Read the model definition and answer for the solid it produces. Units are mm, in the model's axes. A direction names the side the tool comes from. Coordinates: 2 decimals unless noted, no trailing zeros. Order: outer loops, then holes, each group sorted by start corner. A loop starts at its lowest first (then second) coordinate and runs counter-clockwise, first axis right, second up. Notation, with made-up numbers: (52.5, 0.5) -> (96.5, 0.5) arc R31 cw to (96.5, 31.5) -> close; hole circle Ø8 at (85, 46). An arc over 180 degrees is marked (long way). Answer as a JSON object with one key per item and string values. Group by question number.
1) Section B-B on y = 1 is taken. Determine the outline of the cut face in (x, z).
2) Section C-C on z = 0 is taken. Determine the outline of the cut face in (x, y), and give its area (3 significant figures).
3) Consider L1, parallel to Z at x = 0, y = 3.25; L2, parallel to Y at x = 3, z = -3; L3, parallel to X at y = 1.25, z = 5.5. Determine where each line is inside the solid, lowest interval first.
4) Determine the mould class of faces 3 (the cylindrical face through (3.47, 7.66, 15.62)), 4 (the cylindrical face through (-2.17, 4.56, -9.76)), 5 (the flat face through (0, 12, 0)) for opening direction X: released by +X, released by -X, zero draft, split by the parting line, or undercut.
5) Section D-D on y = 7.5 is taken. Determine the outline of the cut face in (x, z).
6) Section A-A on x = 0 is taken. Determine the outline of the cut face in (y, z).
7) A tool of negligible diameter and unlimited length cuts with its end or side. For faces 1 (the flat face through (-11, 5, 9)), 2 (the flat face through (-5.2, 0, 9.1)), from which of +Z, -Z, +X, -X, +Y, -Y can it reach the whole face along a straight path? Write none if from no direction.
8) Given pin 1 (1 mm diameter, centred on x = -2, y = 3, fed in from +Z); pin 2 (6 mm diameter, centred on x = 1.5, y = 3.5, fed in from -Z); pin 3 (4 mm diameter, centred on y = 2.5, z = 1.5, fed in from -X); pin 4 (1 mm diameter, centred on y = 8, z = 10, fed in from +X), each flat-ended and moving along its own axis, determine where each tip first touches the part or whether it passes through.
from build123d import *

# Parameters (mm, degrees)
FILLET1_R          = 2
SKETCH2_R          = 10
CUT_EXTRUDE1_DEPTH = 9
CHAMFER1_SIZE      = 0.25
CHAMFER2_SIZE      = 0.25


with BuildPart() as part:
    # Sketch1 → Revolve1 (revolve)
    with BuildSketch(Plane.XY):
        Polygon((0, 0), (-14, 0), (-14, 5), (-16, 5), (-16, 12), (0, 12), align=None)
    revolve(axis=Axis((0, 12, 0), (0, -1, 0)))

    # Fillet1
    fillet1_edges = [part.edges().sort_by_distance(p)[0] for p in [
        (16, 12, 0),
    ]]
    fillet(fillet1_edges, radius=FILLET1_R)

    # Sketch2 → Cut-Extrude1 (cut)
    with BuildSketch(Plane.XZ):
        Circle(SKETCH2_R)
    extrude(amount=-CUT_EXTRUDE1_DEPTH, mode=Mode.SUBTRACT)

    # Chamfer1
    chamfer1_edges = [part.edges().sort_by_distance(p)[0] for p in [
        (-10, 0, 0),
        (14, 0, 0),
    ]]
    chamfer(chamfer1_edges, length=CHAMFER1_SIZE)

    # Chamfer2
    chamfer2_edges = [part.edges().sort_by_distance(p)[0] for p in [
        (16, 5, 0),
    ]]
    chamfer(chamfer2_edges, length=CHAMFER2_SIZE)


solid = part.part
Worked answers:
{
 "1": {"outline": "circle Ø28 at (0, 0); hole circle Ø20 at (0, 0)"},
 "2": {"outline": "(-16, 5.25) -> (-15.75, 5) -> (-14, 5) -> (-14, 0.25) -> (-13.75, 0) -> (-10.25, 0) -> (-10, 0.25) -> (-10, 9) -> (10, 9) -> (10, 0.25) -> (10.25, 0) -> (13.75, 0) -> (14, 0.25) -> (14, 5) -> (15.75, 5) -> (16, 5.25) -> (16, 10) arc R2 ccw to (14, 12) -> (-14, 12) arc R2 ccw to (-16, 10) -> close", "area": "182 mm²"},
 "3": {"L1": "z = -14 to -10, 10 to 14", "L2": "y = 9 to 12", "L3": "x = -12.87 to -8.35, 8.35 to 12.87"},
 "4": {"face 3": "split by the parting line", "face 4": "undercut", "face 5": "zero draft"},
 "5": {"outline": "circle Ø32 at (0, 0); hole circle Ø20 at (0, 0)"},
 "6": {"outline": "(0, -13.75) -> (0.25, -14) -> (5, -14) -> (5, -15.75) -> (5.25, -16) -> (10, -16) arc R2 ccw to (12, -14) -> (12, 14) arc R2 ccw to (10, 16) -> (5.25, 16) -> (5, 15.75) -> (5, 14) -> (0.25, 14) -> (0, 13.75) -> (0, 10.25) -> (0.25, 10) -> (9, 10) -> (9, -10) -> (0.25, -10) -> (0, -10.25) -> close"},
 "7": {"face 1": "-Y", "face 2": "+Z, -Z, +X, -X, -Y"},
 "8": {"pin 1": "stops at z = 13.92", "pin 2": "stops at z = -16", "pin 3": "stops at x = -14", "pin 4": "stops at x = 12.87"}
}
